Autodesk Inventor part; units mm, degrees
ref_plane "YZ Plane" through (0, 0, 0) normal (1, 0, 0) x (0, 1, 0)
ref_plane "XZ Plane" through (0, 0, 0) normal (0, 1, 0) x (-1, 0, 0)
ref_plane "XY Plane" through (0, 0, 0) normal (0, 0, 1) x (1, 0, 0)
sketch "Sketch1" plane through (0, 0, 0) normal (0, 0, 1) x (1, 0, 0)
  line L0 (-305, 610) -> (305, 610)
  line L1 (305, 610) -> (305, -610)
  line L2 (305, -610) -> (-305, -610)
  line L3 (-305, -610) -> (-305, 610)
  line L4 (-305, 610) -> (305, -610) construction
  line L5 (305, 610) -> (-305, -610) construction
  point P0 (0, 0)
  dimension "d0" = 610
  dimension "d1" = 1220
extrude "Extrusion1" add sketch "Sketch1" along normal blind 20
sketch "Sketch2" plane through (0, 0, 20) normal (0, 0, 1) x (1, 0, 0)
  circle A0 centre (82.5, 575) radius 5
  circle A1 centre (82.5, -25) radius 5
  circle A2 centre (82.5, 375) radius 5
  circle A3 centre (82.5, -225) radius 5
  circle A4 centre (82.5, 175) radius 5
  arc A5 (92.5, -250) -> (97.5, -245) centre (92.5, -245) ccw
  line L0 (69.5, -250) -> (92.5, -250)
  line L1 (69.5, -250) -> (69.5, 600)
  line L2 (92.5, 600) -> (69.5, 600)
  arc A6 (97.5, 595) -> (92.5, 600) centre (92.5, 595) ccw
  line L3 (97.5, -245) -> (97.5, 595)
  circle A7 centre (-82.5, 575) radius 5
  circle A8 centre (-82.5, -25) radius 5
  circle A9 centre (-82.5, 375) radius 5
  circle A10 centre (-82.5, -225) radius 5
  circle A11 centre (-82.5, 175) radius 5
  arc A12 (-97.5, -245) -> (-92.5, -250) centre (-92.5, -245) ccw
  line L4 (-97.5, 595) -> (-97.5, -245)
  arc A13 (-92.5, 600) -> (-97.5, 595) centre (-92.5, 595) ccw
  line L5 (-69.5, 600) -> (-92.5, 600)
  line L6 (-69.5, -250) -> (-69.5, 600)
  line L7 (-92.5, -250) -> (-69.5, -250)
  point P0 (0, 0)
extrude "Extrusion2" cut sketch "Sketch2" against normal through all contours A0 | A1 | A2 | A3 | A4 | A7 | A8 | A9 | A10 | A11
sketch "Sketch3" plane through (0, 0, 20) normal (0, 0, 1) x (1, 0, 0)
  circle A0 centre (-82.5, 575) radius 5
  point P0 (0, 0)
hole "Hole1" at (-82.5, 575, 20) direction (0, 0, -1) diameter 8 end through all countersink diameter 25 countersink angle 90
mirror "Mirror1" about plane through (0, 0, 0) normal (1, 0, 0) of "Hole1"
pattern_linear "Rectangular Pattern1" count 6 spacing 200 along (0, -1, 0) of "Hole1", "Mirror1"
sketch "Sketch4" plane through (0, 0, 20) normal (0, 0, 1) x (1, 0, 0)
  circle A0 centre (82.5, -425) radius 5
  circle A1 centre (-82.5, -425) radius 5
  point P0 (0, 0)
extrude "Extrusion3" cut sketch "Sketch4" against normal through all
equation "\"BendRadius\" = Thickness"
equation "\"BendReliefWidth\" = Thickness"
equation "\"BendReliefDepth\" = 0.5 * Thickness"
equation "\"CornerReliefSize\" = 4 * Thickness"
equation "\"MinimumRemnant\" = 2 * Thickness"
equation "\"TransitionRadius\" = BendRadius"
equation "\"JacobiRadiusSize\" = Thickness"
equation "\"GapSize\" = Thickness"
properties part number "IMS-00-003" material "Wood (Birch)"
Model file for the job. Use its own axes, mm. Round coordinates to 2 decimals unless told otherwise and drop trailing zeros.
(1) Drill centre lines: line 1 (X direction, y = -425, z = 3); line 2 (X direction, y = 378, z = 11.25). Where is each one in solid material? Low to high.
(2) Pull direction Y, two halves, no side cores. Call faces 1 (the face through (-4, 9, 20)), 2 (the face through (82.74, 380.464, 12.969)), 3 (the face through (84.14, 169.78, 12.97)): released by +Y, released by -Y, zero draft, split by the parting line, or undercut.
(3) Pin check, flat tips, straight feed: pin 1 (11.5 mm diameter, centred on x = 82.5, y = 175, fed in from +Z); pin 2 (16 mm diameter, centred on x = 82.5, y = -25, fed in from +Z); pin 3 (13 mm diameter, centred on x = 82.5, y = -425, fed in from +Z). Stop position of each tip, or through.
Verdict:
1. line 1: x = -305 to -87.5, -77.5 to 77.5, 87.5 to 305
1. line 2: x = -305 to -86.5, -78.5 to 78.5, 86.5 to 305
2. face 1: zero draft
2. face 2: undercut
2. face 3: undercut
3. pin 1: stops at z = 13.25
3. pin 2: stops at z = 15.5
3. pin 3: stops at z = 14
